```python
from build123d import *

# Parameters (mm, degrees)
F0_W   = 8
F0_H   = 8.5
F0_W_2 = 13
F0_H_2 = 11.5
F0_W_3 = 9


with BuildPart() as f1:
    # F0 (on Front) → F1 (revolve)
    with BuildSketch(Plane.XZ):
        Polygon((0, 164), (0, 97.5), (8, 97.5), (8, 109), (8, 164), align=None)
        with Locations((4, 93.25)):
            Rectangle(F0_W, F0_H)
        Polygon((21, 109), (21, 97.5), (30, 97.5), (30, 164), (21, 164), align=None)
        with Locations((14.5, 103.25)):
            Rectangle(F0_W_2, F0_H_2)
        with Locations((14.5, 93.25)):
            Rectangle(F0_W_2, F0_H)
        with Locations((25.5, 93.25)):
            Rectangle(F0_W_3, F0_H)
    revolve(axis=Axis((49, 0, 0), (1, 0, 0)))


solid = f1.part
```
For this review, take the finished solid that the model builds, in its own axes (mm). A direction names the side the tool comes from. Round coordinates to 2 decimals unless told otherwise and drop trailing zeros. Write each loop counter-clockwise with the first axis right and the second up, starting at its lowest first coordinate (ties: lowest second). Pieces come first, ordered by that corner, then holes. Notation, with made-up numbers: (57, 81) -> (98, 81) arc R19 ccw to (98, 115) -> close; hole circle Ø8 at (17, 27.5). An arc over 180 degrees is marked (long way). One line per question, with ' | ' between items. Start each with the question number.
1) Wall thickness on line 1 along Z through (x, y) = (14.5, 0); line 2 along X through (y, z) = (46.5, 142.5): over which ranges is each line inside the solid? List them lowest first.
2) For pin 1 Ø1 at (x, z) = (26.5, -130.5) entering from -Y; pin 2 Ø2 at (x, z) = (25, -4) entering from -Y; pin 3 Ø6 at (x, y) = (4, -130.5) entering from +Z, all flat-tipped, find the tip position at first contact; note any pin that passes through.
3) Machinability: for faces 4 (the flat face through (8, 34, -107)), 5 (the cylindrical face through (15.21, -60.15, -65.597)), which of the approach directions +Z, -Z, +X, -X, +Y, -Y give a long, thin tool a straight path to every point of the face, cutting with its end or side? Answer none if there is none.
4) Add section D-D (y = -131). Write out the cut boundary in (x, z).
5) Add section A-A (y = 0). Write out the cut boundary in (x, z), and give its area (3 significant figures).
6) Mouldability with a two-part tool opening along X and no side actions: class faces 1 (the flat face through (30, 71, -71)), 2 (the cylindrical face through (25, 160, -36)), 3 (the flat face through (21, 34, 107)) as +X half, -X half, draft (parallel to the pull), parting line (faces both ways), or undercut.
7) Add section C-C (x = 15). Write out the cut boundary in (y, z), and give its area (3 significant figures).
Reported:
1) line 1: z = -109 to -89, 89 to 109 | line 2: x = 0 to 8, 21 to 30
2) pin 1: stops at y = -99.98 | pin 2: stops at y = -163.97 | pin 3: stops at z = 103.15
3) face 4: none | face 5: +X, -X
4) outline: (0, -98.67) -> (8, -98.67) -> (8, 98.67) -> (0, 98.67) -> close; (21, -98.67) -> (30, -98.67) -> (30, 98.67) -> (21, 98.67) -> close
5) outline: (0, -164) -> (8, -164) -> (8, -109) -> (21, -109) -> (21, -164) -> (30, -164) -> (30, -89) -> (0, -89) -> close; (0, 89) -> (30, 89) -> (30, 164) -> (21, 164) -> (21, 109) -> (8, 109) -> (8, 164) -> (0, 164) -> close | area: 3,070 mm²
6) face 1: +X half | face 2: draft | face 3: undercut
7) outline: circle Ø218 at (0, 0); hole circle Ø178 at (0, 0) | area: 12,400 mm²
